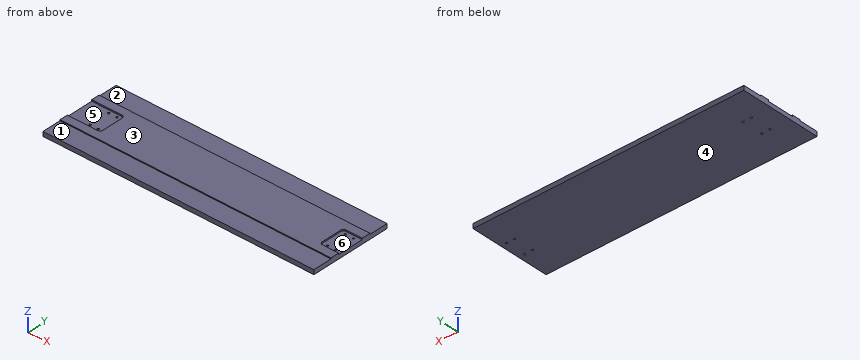
from build123d import *

# Parameters (mm, degrees)
SZKIC1_W                       = 600
SZKIC1_H                       = 180
DODANIE_WYCI_GNI_CIE1_DEPTH    = 10
SZKIC2_W                       = 600
SZKIC2_H                       = 96
DODANIE_WYCI_GNI_CIE2_DEPTH    = 2
SZKIC3_W                       = 42
SZKIC3_H                       = 58
SZKIC3_W_2                     = 73
SZKIC3_H_2                     = 60
WYTNIJ_WYCI_GNI_CIE1_DEPTH     = 3
ZAOKR_GLENIE1_R                = 6
OTW_R_GWINTOWANY_M5X0_82_D     = 4.2
OTW_R_GWINTOWANY_M5X0_83_D     = 4.2
OTW_R_GWINTOWANY_M5X0_83_DEPTH = 17
OTW_R_GWINTOWANY_M5X0_83_TIP   = 1.2618073


with BuildPart() as part:
    # Szkic1 → Dodanie-wyciągnięcie1 (new body)
    with BuildSketch(Plane.XY):
        with Locations((300, 360)):
            Rectangle(SZKIC1_W, SZKIC1_H)
    extrude(amount=DODANIE_WYCI_GNI_CIE1_DEPTH)

    # Szkic2 → Dodanie-wyciągnięcie2 (add)
    with BuildSketch(Plane.XY.offset(10)):
        with Locations((300, 360)):
            Rectangle(SZKIC2_W, SZKIC2_H)
    extrude(amount=DODANIE_WYCI_GNI_CIE2_DEPTH)

    # Szkic3 → Wytnij-wyciągnięcie1 (cut)
    with BuildSketch(Plane.XY.offset(12)):
        with Locations((579, 360)):
            Rectangle(SZKIC3_W, SZKIC3_H)
        with Locations((36.5, 360)):
            Rectangle(SZKIC3_W_2, SZKIC3_H_2)
    extrude(amount=-WYTNIJ_WYCI_GNI_CIE1_DEPTH, mode=Mode.SUBTRACT)

    # Zaokrąglenie1
    zaokr_glenie1_edges = [part.edges().sort_by_distance(p)[0] for p in [
        (73, 390, 10.5),
        (73, 330, 10.5),
        (558, 331, 10.5),
        (558, 389, 10.5),
    ]]
    fillet(zaokr_glenie1_edges, radius=ZAOKR_GLENIE1_R)

    # Otwór gwintowany M5x0.82 (through all)
    with Locations(Plane.XY.offset(9)):
        with Locations((62, 383), (44, 383), (62, 337), (44, 337)):
            Hole(OTW_R_GWINTOWANY_M5X0_82_D / 2)

    # Otwór gwintowany M5x0.83
    with Locations(Plane.XY.offset(9)):
        with Locations((587, 382), (569, 382), (569, 338), (587, 338)):
            Hole(OTW_R_GWINTOWANY_M5X0_83_D / 2, depth=OTW_R_GWINTOWANY_M5X0_83_DEPTH)
            with Locations((0, 0, -(OTW_R_GWINTOWANY_M5X0_83_DEPTH + OTW_R_GWINTOWANY_M5X0_83_TIP / 2))):  # 118° drill point
                Cone(0, OTW_R_GWINTOWANY_M5X0_83_D / 2, OTW_R_GWINTOWANY_M5X0_83_TIP, mode=Mode.SUBTRACT)


solid = part.part
Read the model definition and answer for the solid it produces. Units are mm, in the model's axes. Face numbers are marked on the shaded views. A direction names the side the tool comes from. Round coordinates to 2 decimals unless told otherwise and drop trailing zeros. Order: outer loops, then holes, each group sorted by start corner. A loop starts at its lowest first (then second) coordinate and runs counter-clockwise, first axis right, second up. Notation, with made-up numbers: (12.5, -16) - (18.5, -16) arc R20 ccw to (18.5, -12) - close; hole circle Ø6 at (-6.5, -27.5). An arc over 180 degrees is marked (long way). Use one line per item in the form item = value. Start each with the question number.
(1) Find the intervals of material crossed by line 1 along Y through (x, z) = (44, 2.25); line 2 along Y through (x, z) = (587, 4.25); line 3 along X through (y, z) = (337, 3.25), in increasing order. Write a range as from..to.
(2) Determine the mould class of the marked faces 4, 5 and 6 for opening direction Y: +Y half, -Y half, draft (parallel to the pull), parting line (faces both ways), or undercut.
(3) For the marked faces 1, 2 and 3, determine the directions among +Z, -Z, +X, -X, +Y, -Y from which every point of the face is accessible in a straight line to the end or side of a thin tool.
(4) The part is cut by section A-A (x = 447.5). Give the vertices of the cut face in (y, z).
(5) Flat-ended cylindrical pins translate along their axes: pin 1 Ø0.9 at (x, z) = (584.5, 10.5) entering from +Y; pin 2 Ø0.6 at (x, z) = (239, 11.5) entering from -Y; pin 3 Ø0.9 at (y, z) = (354, 10) entering from -X; pin 4 Ø4 at (x, y) = (44, 383) entering from +Z. Find the tip coordinate at first contact, or state that the pin passes through.
(6) The part is cut by section B-B (y = 301.5). Give the vertices of the cut face in (x, z).
Checked values:
q1.line_1 = 270..334.9, 339.1..380.9, 385.1..450
q1.line_2 = 270..335.9, 340.1..379.9, 384.1..450
q1.line_3 = 0..41.9, 46.1..59.9, 64.1..567.15, 570.85..585.15, 588.85..600
q2.face_4 = draft
q2.face_5 = undercut
q2.face_6 = undercut
q3.face_1 = +Z, +X, -X, -Y
q3.face_2 = +Z, +X, -X, +Y
q3.face_3 = +Z, +X, -X, +Y, -Y
q4.outline = (270, 0) - (450, 0) - (450, 10) - (408, 10) - (408, 12) - (312, 12) - (312, 10) - (270, 10) - close
q5.pin_1 = 408
q5.pin_2 = 312
q5.pin_3 = 73
q5.pin_4 = through
q6.outline = (0, 0) - (600, 0) - (600, 10) - (0, 10) - close
